Could you check a few things on this model? Use its own coordinates, in mm. A direction names the side the tool comes from. Coordinates: 2 decimals unless noted, no trailing zeros. Order: outer loops, then holes, each group sorted by start corner. A loop starts at its lowest first (then second) coordinate and runs counter-clockwise, first axis right, second up. Notation, with made-up numbers: (37, -8) - (82, -8) arc R18 cw to (82, 21) - close; hole circle Ø1 at (-30, 1.25). An arc over 180 degrees is marked (long way). Answer as a JSON object with one key per item and string values. Group by question number.
(1) Imagine slicing it at C-C, the plane x = -1. Write out the boundary of the cut face in (y, z), and give its area (3 significant figures).
(2) Imagine slicing it at B-B, the plane z = 17.75. Write out the boundary of the cut face in (x, y) (3 decimals).
(3) Imagine slicing it at D-D, the plane y = 5. Write out the boundary of the cut face in (x, z), and give its area (3 significant figures).
(4) Please list where these lines run through material, in increasing order: probe 1 along Z at (x, y) = (-6.75, 1.2) (3 decimals); probe 2 along Z at (x, y) = (6.75, 1.4) (3 decimals); probe 3 along Z at (x, y) = (1.5, 5).
(5) Will these pins go through, and if not, where does the flat tip stop? P1, Ø4, axis at x = 6.5, y = 5, coming from the +Z side; P2, Ø3.5, axis at x = 6.75, z = 24.55, coming from the +Y side; P3, Ø2.5, axis at x = 6.75, z = 17.75, coming from the -Y side; P4, Ø10, axis at x = 8, z = 9, coming from the +Y side.
(6) Which directions (+Z, -Z, +X, -X, +Y, -Y) give clear straight access to the entire face, cutting with the end or side of a thin tool? Please do faces 1 (the cylindrical face through (-0.16, 1.26, -1.11)), 2 (the flat face through (0, 2, 18)).
(7) Imagine slicing it at A-A, the plane x = -6.75. Write out the boundary of the cut face in (y, z) (3 decimals), and give its area (3 significant figures).
(8) We'd pull the mould along Z, two halves only. Please class faces 3 (the cylindrical face through (0.165, 2.502, 0.088)), 4 (the cylindrical face through (0.165, 2.752, 3.713)), 5 (the flat face through (11.75, 1, 11)): pulls with the +Z half, pulls with the -Z half, needs draft (parallel to the pull), parting line crosses it, or undercut.
from build123d import *

# Parameters (mm, degrees)
SKETCH1_W           = 23.5
SKETCH1_H           = 2
BOSS_EXTRUDE1_DEPTH = 30
SKETCH2_R           = 3
SKETCH2_R_2         = 2
BOSS_EXTRUDE2_DEPTH = 23.5
FILLET1_R           = 110
FILLET2_R           = 2.5
SKETCH3_R           = 1.125
CUT_EXTRUDE1_DEPTH  = 24


with BuildPart() as part:
    # Sketch1 → Boss-Extrude1 (new body)
    with BuildSketch(Plane.XY):
        with Locations((0, 1)):
            Rectangle(SKETCH1_W, SKETCH1_H)
    extrude(amount=BOSS_EXTRUDE1_DEPTH)

    # Sketch2 → Boss-Extrude2 (add)
    with BuildSketch(Plane(origin=(11.75, 0, 0), x_dir=(0, 0, -1), z_dir=(1, 0, 0))):
        with Locations((0, 4.5)):
            Circle(SKETCH2_R)
        with Locations(Location((0, 4.5, 0), (0, 0, 90))):
            Circle(SKETCH2_R_2, mode=Mode.SUBTRACT)
    extrude(amount=-BOSS_EXTRUDE2_DEPTH)

    # Fillet1
    # the kernel refuses this fillet: 110 mm, written as the material it adds along each edge
    with BuildSketch(Plane(origin=(-11.75, 1.5, 0), x_dir=(0, -1, 0), z_dir=(1, 0, 0))) as fillet1_piece_1:
        with BuildLine():
            CenterArc((73.583333333, 83.090270523), FILLET1_R, 227.333597139, 1.723771549)
            ThreePointArc((-0.966814159, 2.205936386), (-0.252313926, 1.204251319), (0, 0))
            Line((0, 0), (1.5, 0))
        make_face()
    extrude(amount=23.5)

    # Fillet2
    fillet2_edges = [part.edges().sort_by_distance(p)[0] for p in [
        (0, 2, 1.658312395),
    ]]
    fillet(fillet2_edges, radius=FILLET2_R)

    # Sketch3 → Cut-Extrude1 (cut)
    with BuildSketch(Plane(origin=(0, 2, 0), x_dir=(1, 0, 0), z_dir=(0, 1, 0))):
        with Locations(Location((-6.75, -10.95, 0), (0, 0, 180))):
            Circle(SKETCH3_R)
        with Locations(Location((-6.75, -17.75, 0), (0, 0, 180))):
            Circle(SKETCH3_R)
        with Locations(Location((-6.75, -24.55, 0), (0, 0, 180))):
            Circle(SKETCH3_R)
        with Locations(Location((6.75, -24.55, 0), (0, 0, 180))):
            Circle(SKETCH3_R)
        with Locations(Location((6.75, -17.75, 0), (0, 0, 180))):
            Circle(SKETCH3_R)
        with Locations(Location((6.75, -10.95, 0), (0, 0, 180))):
            Circle(SKETCH3_R)
    extrude(amount=-CUT_EXTRUDE1_DEPTH, mode=Mode.SUBTRACT)


solid = part.part
Result set:
{
 "1": {"outline": "(0, 0) arc R110 cw to (2.47, -2.21) arc R3 ccw (long way) to (4.5, 3) arc R2.5 cw to (2, 5.5) - (2, 30) - (0, 30) - close; hole circle Ø4 at (4.5, 0)", "area": "78.7 mm^2"},
 "2": {"outline": "(-11.75, 0) - (-7.875, 0) - (-7.875, 2) - (-11.75, 2) - close; (-5.625, 0) - (5.625, 0) - (5.625, 2) - (-5.625, 2) - close; (7.875, 0) - (11.75, 0) - (11.75, 2) - (7.875, 2) - close"},
 "3": {"outline": "(-11.75, -2.96) - (11.75, -2.96) - (11.75, -1.94) - (-11.75, -1.94) - close; (-11.75, 1.94) - (11.75, 1.94) - (11.75, 2.96) - (-11.75, 2.96) - close", "area": "48.0 mm^2"},
 "4": {"probe 1": "z = -1.056 to 9.825, 12.075 to 16.625, 18.875 to 23.425, 25.675 to 30", "probe 2": "z = -1.236 to 9.825, 12.075 to 16.625, 18.875 to 23.425, 25.675 to 30", "probe 3": "z = -2.96 to -1.94, 1.94 to 2.96"},
 "5": {"P1": "stops at z = 3.5", "P2": "stops at y = 2", "P3": "stops at y = 0", "P4": "stops at y = 2.5"},
 "6": {"face 1": "-Z, +X, -X, -Y", "face 2": "+Z, +X, -X, +Y"},
 "7": {"outline": "(0, 0) arc R110 cw to (2.467, -2.206) arc R3 ccw (long way) to (4.5, 3) arc R2.5 cw to (2, 5.5) - (2, 9.825) - (0, 9.825) - close; (0, 12.075) - (2, 12.075) - (2, 16.625) - (0, 16.625) - close; (0, 18.875) - (2, 18.875) - (2, 23.425) - (0, 23.425) - close; (0, 25.675) - (2, 25.675) - (2, 30) - (0, 30) - close; hole circle Ø4 at (4.5, 0)", "area": "65.2 mm^2"},
 "8": {"face 3": "undercut", "face 4": "pulls with the +Z half", "face 5": "needs draft"}
}
